Verification items for the finished model (mm, model axes). A direction names the side the tool comes from. Coordinates: 2 decimals unless noted, no trailing zeros. Order: outer loops, then holes, each group sorted by start corner. A loop starts at its lowest first (then second) coordinate and runs counter-clockwise, first axis right, second up. Notation, with made-up numbers: M -6,-21.5 L 32,-21.5 A17 ccw 32,-17.5 Z; hole C -34.75,62 d5. An arc over 180 degrees is marked long. Return JSON: item names as keys, results as strings.
```python
from build123d import *

# Parameters (mm, degrees)
BOSS_EXTRUDE1_DEPTH = 35
CUT_EXTRUDE1_DEPTH  = 26
SKETCH4_W           = 36.590571665
SKETCH4_H           = 16.65
BOSS_EXTRUDE2_DEPTH = 4.3
SKETCH5_W           = 22.6
SKETCH5_H           = 11.85
CUT_EXTRUDE2_DEPTH  = 4.2
CUT_EXTRUDE3_DEPTH  = 17.2
BOSS_EXTRUDE3_DEPTH = 23
SKETCH11_R          = 1.5625
CUT_EXTRUDE7_DEPTH  = 12.54
SKETCH13_R          = 1.7526
CUT_EXTRUDE8_DEPTH  = 16
SKETCH15_W          = 11
SKETCH15_H          = 18.91
BOSS_EXTRUDE4_DEPTH = 22


with BuildPart() as part:
    # Sketch1 → Boss-Extrude1 (new body)
    with BuildSketch(Plane.XY):
        Polygon((0, 50.21875), (0, 0), (82, 0), (82, 60), (44.352804008, 60), (37.500008496, 71.86939), (12.500002832, 71.86939), align=None)
    extrude(amount=BOSS_EXTRUDE1_DEPTH)

    # Sketch3 → Cut-Extrude1 (cut)
    with BuildSketch(Plane.XY.offset(35)):
        Polygon((42.909428335, 57.5), (36.056632823, 69.36939), (13.943378505, 69.36939), (2.5, 49.548877019), (2.5, 2.5), (79.5, 2.5), (79.5, 57.5), align=None)
    extrude(amount=-CUT_EXTRUDE1_DEPTH, mode=Mode.SUBTRACT)

    # Sketch4 → Boss-Extrude2 (add)
    with BuildSketch(Plane.XY.offset(9)):
        with Locations((61.204714168, 49.175)):
            Rectangle(SKETCH4_W, SKETCH4_H)
    extrude(amount=BOSS_EXTRUDE2_DEPTH)

    # Sketch5 → Cut-Extrude2 (cut)
    with BuildSketch(Plane.XY.offset(13.3)):
        with Locations((60.82763, 51.575)):
            Rectangle(SKETCH5_W, SKETCH5_H)
    extrude(amount=-CUT_EXTRUDE2_DEPTH, mode=Mode.SUBTRACT)

    # Sketch6 → Cut-Extrude3 (cut)
    with BuildSketch(Plane.XY.offset(9.1)):
        with BuildLine():
            Line((61.72763, 54.15), (60.723855071, 54.15))
            ThreePointArc((60.723855071, 54.15), (49.52763, 51.55), (60.723855071, 48.95))
            Line((60.723855071, 48.95), (61.72763, 48.95))
            ThreePointArc((61.72763, 48.95), (64.32763, 51.55), (61.72763, 54.15))
        make_face()
    extrude(amount=-CUT_EXTRUDE3_DEPTH, mode=Mode.SUBTRACT)

    # Sketch7 → Boss-Extrude3 (add)
    with BuildSketch(Plane.XY.offset(9)):
        Polygon((40.909428335, 56.964101615), (40.909428335, 54.429795973), (42.909428335, 54.429795973), (42.909428335, 57.5), (36.056632823, 69.36939), (13.943378505, 69.36939), (2.5, 49.548877019), (2.5, 2.5), (79.5, 2.5), (79.5, 40.85), (77.5, 40.85), (77.5, 4.5), (4.5, 4.5), (4.5, 49.012978634), (15.098079043, 67.36939), (34.901932285, 67.36939), align=None)
    extrude(amount=BOSS_EXTRUDE3_DEPTH)

    # Sketch11 → Cut-Extrude7 (cut)
    with BuildSketch(Plane.XY.offset(9)):
        with BuildLine():
            Line((6.14367659, 51.85991), (8.89, 51.85991))
            ThreePointArc((8.89, 51.85991), (12.1205, 48.62941), (8.89, 45.39891))
            Line((8.89, 45.39891), (4.5, 45.39891))
            Line((4.5, 45.39891), (4.5, 12.1205))
            Line((4.5, 12.1205), (8.89, 12.1205))
            ThreePointArc((8.89, 12.1205), (11.174308457, 11.174308457), (12.1205, 8.89))
            Line((12.1205, 8.89), (12.1205, 4.5))
            Line((12.1205, 4.5), (35.398460219, 4.5))
            Line((35.398460219, 4.5), (35.398460219, 9.237253753))
            ThreePointArc((35.398460219, 9.237253753), (36.826407652, 13.014445691), (40.396010976, 14.90234))
            Line((40.396010976, 14.90234), (72.25, 14.90234))
            Line((72.25, 14.90234), (72.25, 30.90234))
            Line((72.25, 30.90234), (42.909428335, 30.90234))
            Line((42.909428335, 30.90234), (42.909428335, 54.429795973))
            Line((42.909428335, 54.429795973), (40.909428335, 54.429795973))
            Line((40.909428335, 54.429795973), (40.909428335, 56.964101615))
            Line((40.909428335, 56.964101615), (34.901932285, 67.36939))
            Line((34.901932285, 67.36939), (15.098079043, 67.36939))
            Line((15.098079043, 67.36939), (6.14367659, 51.85991))
        make_face()
        with Locations((8.89, 8.89)):
            Circle(SKETCH11_R)
        with Locations((8.89, 48.62941)):
            Circle(SKETCH11_R)
        with Locations((41.108128667, 9.237253753)):
            Circle(SKETCH11_R)
    extrude(amount=-CUT_EXTRUDE7_DEPTH, mode=Mode.SUBTRACT)

    # Sketch13 → Cut-Extrude8 (cut)
    with BuildSketch(Plane.XY.offset(9)):
        with Locations((60.00821, 11)):
            Circle(SKETCH13_R)
        with Locations((60.00821, 35)):
            Circle(SKETCH13_R)
    extrude(amount=-CUT_EXTRUDE8_DEPTH, mode=Mode.SUBTRACT)

    # Sketch15 → Boss-Extrude4 (add)
    with BuildSketch(Plane(origin=(0, 0, 0), x_dir=(-1, 0, 0), z_dir=(0, 0, -1))):
        with Locations((-25, 13.955)):
            Rectangle(SKETCH15_W, SKETCH15_H)
    extrude(amount=-BOSS_EXTRUDE4_DEPTH)


solid = part.part
```
Q1. Cross-section at A-A, the plane x = 31.5. Record the boundary of the cut face in (y, z).
Values:
{"outline": "M 0,0 L 4.5,0 L 4.5,32 L 2.5,32 L 2.5,35 L 0,35 Z; M 67.37,0 L 71.87,0 L 71.87,35 L 69.37,35 L 69.37,32 L 67.37,32 Z"}
Q2. Cross-section at B-B, the plane z = 30. Record the boundary of the cut face in (x, y).
Values:
{"outline": "M 0,0 L 82,0 L 82,60 L 44.35,60 L 37.5,71.87 L 12.5,71.87 L 0,50.22 Z; hole M 4.5,4.5 L 77.5,4.5 L 77.5,40.85 L 79.5,40.85 L 79.5,57.5 L 42.91,57.5 L 42.91,54.43 L 40.91,54.43 L 40.91,56.96 L 34.9,67.37 L 15.1,67.37 L 4.5,49.01 Z"}
Q3. Go/stop test with flat-tipped pins: pin 1 (6 mm diameter, centred on x = 55, y = 19.5, fed in from +Z); pin 2 (2 mm diameter, centred on x = 58.5, z = 11.5, fed in from +Y); pin 3 (4.5 mm diameter, centred on x = 54, y = 48, fed in from +Z); pin 4 (4 mm diameter, centred on x = 60.01, y = 35, fed in from +Z). Record where each tip stops, or that it passes through.
Values:
{"pin 1": "through", "pin 2": "y = 60", "pin 3": "z = 9.1", "pin 4": "z = 9"}
Q4. Material ranges on line 1 along X through (y, z) = (6.5, 16); line 2 along Y through (x, z) = (77, 30); line 3 along X through (y, z) = (5.5, 32.5), recorded low to high.
Values:
{"line 1": "0 to 4.5, 19.5 to 30.5, 77.5 to 82", "line 2": "0 to 4.5, 57.5 to 60", "line 3": "0 to 2.5, 79.5 to 82"}
Q5. Cross-section at C-C, the plane z = 10.5. Record the boundary of the cut face in (x, y).
Values:
{"outline": "M 0,0 L 82,0 L 82,60 L 44.35,60 L 37.5,71.87 L 12.5,71.87 L 0,50.22 Z; hole M 4.5,4.5 L 19.5,4.5 L 19.5,23.41 L 30.5,23.41 L 30.5,4.5 L 77.5,4.5 L 77.5,40.85 L 42.91,40.85 L 42.91,54.43 L 40.91,54.43 L 40.91,56.96 L 34.9,67.37 L 15.1,67.37 L 4.5,49.01 Z; hole M 49.53,45.65 L 72.13,45.65 L 72.13,57.5 L 49.53,57.5 Z"}
Q6. Draft check along Y on faces 1 (the face through (40, 0, 17)), 2 (the face through (58, 30.902, 5)), 3 (the face through (40.974, 65.852, 17.255)). Enter one of: pulls with the +Y half, pulls with the -Y half, needs draft (parallel to the pull), parting line crosses it, or undercut.
Values:
{"face 1": "pulls with the -Y half", "face 2": "undercut", "face 3": "pulls with the +Y half"}
Q7. Tool access check on faces 4 (the face through (42.909, 43, 5)), 5 (the face through (0, 25, 17)), 6 (the face through (77.5, 23, 20)). Record the directions out of +Z, -Z, +X, -X, +Y, -Y that give a thin tool (end or side, any length) a straight path to the whole face; none if there is none.
Values:
{"face 4": "+Z, -Z", "face 5": "+Z, -Z, -X, +Y, -Y", "face 6": "+Z"}
Q8. Cross-section at D-D, the plane x = 74. Record the boundary of the cut face in (y, z).
Values:
{"outline": "M 0,0 L 60,0 L 60,35 L 57.5,35 L 57.5,13.3 L 40.85,13.3 L 40.85,9 L 4.5,9 L 4.5,32 L 2.5,32 L 2.5,35 L 0,35 Z"}
